Can you work these out from the model? Positions are in its coordinate system, mm. A direction names the side the tool comes from. Round coordinates to 2 decimals unless told otherwise and drop trailing zeros. Loops run counter-clockwise (first coordinate to the right, second up) from the corner with the lowest first, then second, coordinate; pieces in that order, holes last. Notation, with made-up numbers: M 8.25,-40 L 17.25,-40 A3 ccw 17.25,-36 Z; hole C 41,-25.75 d4. An arc over 180 degrees is marked long. Use a Markdown table: item, result. Add a question column.
```python
from build123d import *

# Parameters (mm, degrees)
EXTRUDE_1_DEPTH     = 75
SHELL_1_T           = -2
SKETCH_2_R          = 23.5
CUT_EXTRUDE_1_DEPTH = 194.70352352


with BuildPart() as part:
    # 草图1 → 凸台-拉伸1 (new, symmetric)
    with BuildSketch(Plane(origin=(0, 0, 0), x_dir=(0, 0, -1), z_dir=(1, 0, 0))):
        Polygon((0, 0), (85, 0), (85, -30), (26.704728189, -88.295271811), (-26.704728189, -88.295271811), (-85, -30), (-85, 0), align=None)
    extrude(amount=EXTRUDE_1_DEPTH, both=True)

    # 抽壳1
    shell_1_openings = [part.faces().sort_by_distance(p)[0] for p in [
        (0, 0, 0),
        (0, -88.295271811, 0),
    ]]
    offset(amount=SHELL_1_T, openings=shell_1_openings, kind=Kind.INTERSECTION)

    # 草图2 → 切除-拉伸1 (cut, through all)
    with BuildSketch(Plane(origin=(75, 0, 0), x_dir=(0, 0, -1), z_dir=(1, 0, 0))):
        with Locations((0, -88.295271811)):
            Circle(SKETCH_2_R)
    extrude(amount=-CUT_EXTRUDE_1_DEPTH, mode=Mode.SUBTRACT)


solid = part.part
```
(1) On a 3-axis mill with a long thin cutter (end or side, diameter ignored), from which of +Z, -Z, +X, -X, +Y, -Y can I reach the whole of each face in a straight line? I mean faces 1 (the face through (1.02, -58.32, -53.85)), 2 (the face through (-74, -64.8, -0.5)). Say none if no direction works.
(2) Suppose I cut it at A-A on z = 0. List the corners of the cut face in (x, y) for me, and give its area (3 significant figures).
(3) Suppose I cut it at C-C on y = -75. List the corners of the cut face in (x, z) for me, and give its area (3 significant figures).
(4) I'm going to push a flat-ended pin straight in: pin 1 (2 mm diameter, centred on x = -22, y = -45.5, fed in from +Z). Where does the tip first touch, or does it pass through?
(5) Suppose I cut it at D-D on y = -21. List the corners of the cut face in (x, z) for me, and give its area (3 significant figures).
(6) If I drill on probe 1 along X at (y, z) = (-9.5, 34); probe 2 along Z at (x, y) = (-63.5, -10); probe 3 along Z at (x, y) = (1.5, -47.5), over which ranges is the centre line in solid material (lowest first)? Write a range as [from, to].
(7) Suppose I cut it at B-B on x = -38.5. List the corners of the cut face in (y, z) for me, and give its area (3 significant figures).
(8) Thinking about a two-plate mould opening in Z: for faces 3 (the face through (-73, -34, -1)), 4 (the face through (-75, -34, -1)), 5 (the face through (1, -14, -83)), 6 (the face through (1, -15, 85)), which applies, released by +Z, released by -Z, zero draft, split by the parting line, or undercut?
Results below:
| question | item | result |
|---|---|---|
| 1 | face 1 | +Y |
| 1 | face 2 | +X, -X, -Y |
| 2 | outline | M -75,-64.8 L -73,-64.8 L -73,0 L -75,0 Z; M 73,-64.8 L 75,-64.8 L 75,0 L 73,0 Z |
| 2 | area | 259 mm² |
| 3 | outline | M -75,-40 L 75,-40 L 75,-19.38 L 73,-19.38 L 73,-37.17 L -73,-37.17 L -73,-19.38 L -75,-19.38 Z; M -75,19.38 L -73,19.38 L -73,37.17 L 73,37.17 L 73,19.38 L 75,19.38 L 75,40 L -75,40 Z |
| 3 | area | 991 mm² |
| 4 | pin 1 | stops at z = 70.5 |
| 5 | outline | M -75,-85 L 75,-85 L 75,85 L -75,85 Z; hole M -73,-83 L 73,-83 L 73,83 L -73,83 Z |
| 5 | area | 1,260 mm² |
| 6 | probe 1 | x = [-75, -73], [73, 75] |
| 6 | probe 2 | z = [-85, -83], [83, 85] |
| 6 | probe 3 | z = [-67.5, -64.67], [64.67, 67.5] |
| 7 | outline | M -88.3,-26.7 L -30,-85 L 0,-85 L 0,-83 L -29.17,-83 L -88.3,-23.88 Z; M -88.3,23.88 L -29.17,83 L 0,83 L 0,85 L -30,85 L -88.3,26.7 Z |
| 7 | area | 450 mm² |
| 8 | face 3 | undercut |
| 8 | face 4 | zero draft |
| 8 | face 5 | undercut |
| 8 | face 6 | released by +Z |
